Part model, mm, in its own coordinate system. Round coordinates to 2 decimals unless told otherwise and drop trailing zeros. Loops run counter-clockwise (first coordinate to the right, second up) from the corner with the lowest first, then second, coordinate; pieces in that order, holes last. Notation, with made-up numbers: M 79,69 L 124,69 A19 cw 124,91 Z; hole C -9.75,37 d10. An arc over 180 degrees is marked long. Put each result on its own line as item: value. Start each with the question number.
```python
from build123d import *

# Parameters (mm, degrees)
SKETCH1_W           = 127
SKETCH1_H           = 101.6
BOSS_EXTRUDE1_DEPTH = 1.27
CUT_EXTRUDE1_REACH  = 83.33
SKETCH2_W           = 6.35
SKETCH2_H           = 9.525
CUT_EXTRUDE2_REACH  = 83.33
SKETCH3_W           = 11.1125
SKETCH3_H           = 17.4625


with BuildPart() as part:
    # Sketch1 → Boss-Extrude1 (new body)
    with BuildSketch(Plane(origin=(0, 0, 0), x_dir=(1, 0, 0), z_dir=(0, 1, 0))):
        Rectangle(SKETCH1_W, SKETCH1_H)
    extrude(amount=BOSS_EXTRUDE1_DEPTH)

    # Sketch2 → Cut-Extrude1 (cut, up to next)
    with BuildSketch(Plane(origin=(0, 1.27, 0), x_dir=(1, 0, 0), z_dir=(0, 1, 0)), mode=Mode.PRIVATE) as cut_extrude1_sk1:
        with Locations((-56.515, 42.2275)):
            Rectangle(SKETCH2_W, SKETCH2_H)
    cut_extrude1_tool1 = extrude(cut_extrude1_sk1.sketch, amount=-CUT_EXTRUDE1_REACH, mode=Mode.PRIVATE) & part.part
    # Sketch2 → Cut-Extrude1 (cut, up to next)
    with BuildSketch(Plane(origin=(0, 1.27, 0), x_dir=(1, 0, 0), z_dir=(0, 1, 0)), mode=Mode.PRIVATE) as cut_extrude1_sk2:
        with Locations((56.515, 42.2275)):
            Rectangle(SKETCH2_W, SKETCH2_H)
    cut_extrude1_tool2 = extrude(cut_extrude1_sk2.sketch, amount=-CUT_EXTRUDE1_REACH, mode=Mode.PRIVATE) & part.part
    # Sketch2 → Cut-Extrude1 (cut, up to next)
    with BuildSketch(Plane(origin=(0, 1.27, 0), x_dir=(1, 0, 0), z_dir=(0, 1, 0)), mode=Mode.PRIVATE) as cut_extrude1_sk3:
        with Locations((56.515, -42.2275)):
            Rectangle(SKETCH2_W, SKETCH2_H)
    cut_extrude1_tool3 = extrude(cut_extrude1_sk3.sketch, amount=-CUT_EXTRUDE1_REACH, mode=Mode.PRIVATE) & part.part
    # Sketch2 → Cut-Extrude1 (cut, up to next)
    with BuildSketch(Plane(origin=(0, 1.27, 0), x_dir=(1, 0, 0), z_dir=(0, 1, 0)), mode=Mode.PRIVATE) as cut_extrude1_sk4:
        with Locations((-56.515, -42.2275)):
            Rectangle(SKETCH2_W, SKETCH2_H)
    cut_extrude1_tool4 = extrude(cut_extrude1_sk4.sketch, amount=-CUT_EXTRUDE1_REACH, mode=Mode.PRIVATE) & part.part
    add(cut_extrude1_tool1.solids().sort_by_distance((-56.515, 1.27, -42.2275))[0], mode=Mode.SUBTRACT)
    add(cut_extrude1_tool2.solids().sort_by_distance((56.515, 1.27, -42.2275))[0], mode=Mode.SUBTRACT)
    add(cut_extrude1_tool3.solids().sort_by_distance((56.515, 1.27, 42.2275))[0], mode=Mode.SUBTRACT)
    add(cut_extrude1_tool4.solids().sort_by_distance((-56.515, 1.27, 42.2275))[0], mode=Mode.SUBTRACT)

    # Sketch3 → Cut-Extrude2 (cut, up to next)
    with BuildSketch(Plane(origin=(0, 1.27, 0), x_dir=(1, 0, 0), z_dir=(0, 1, 0)), mode=Mode.PRIVATE) as cut_extrude2_sk1:
        with Locations((37.30625, 0)):
            Rectangle(SKETCH3_W, SKETCH3_H)
    cut_extrude2_tool1 = extrude(cut_extrude2_sk1.sketch, amount=-CUT_EXTRUDE2_REACH, mode=Mode.PRIVATE) & part.part
    add(cut_extrude2_tool1.solids().sort_by_distance((37.30625, 1.27, 0))[0], mode=Mode.SUBTRACT)


solid = part.part
```
1. Cut at C-C, the plane z = 3.5. Give the cut face in (x, y), and give its area (3 significant figures).
2. Wall check: L1, parallel to X at y = 1.05, z = 40; L2, parallel to Z at x = -54.5, y = 0.2 (3 decimals); L3, parallel to X at y = 1.15, z = 4. Give the ranges that are in metal, low to high.
3. Cut at A-A, the plane z = -39. Give the cut face in (x, y), and give its area (3 significant figures).
4. Cut at B-B, the plane y = 0.95. Give the number of separate pieces and of enclosed holes in the cut face, and give its area (3 significant figures).
Results list:
1. outline: M -63.5,0 L 31.75,0 L 31.75,1.27 L -63.5,1.27 Z; M 42.86,0 L 63.5,0 L 63.5,1.27 L 42.86,1.27 Z
1. area: 147 mm^2
2. L1: x = -63.5 to -59.69, -53.34 to 53.34, 59.69 to 63.5
2. L2: z = -50.8 to -46.99, -37.465 to 37.465, 46.99 to 50.8
2. L3: x = -63.5 to 31.75, 42.86 to 63.5
3. outline: M -63.5,0 L -59.69,0 L -59.69,1.27 L -63.5,1.27 Z; M -53.34,0 L 53.34,0 L 53.34,1.27 L -53.34,1.27 Z; M 59.69,0 L 63.5,0 L 63.5,1.27 L 59.69,1.27 Z
3. area: 145 mm^2
4. separate pieces: 1
4. enclosed holes: 5
4. area: 12,500 mm^2
